Could you check a few things on this drawing? It's one solid part, dimensions in mm from its lowest x, y, z. A direction names the side the tool comes from. Coordinates: 2 decimals unless noted, no trailing zeros. Write each loop counter-clockwise with the first axis right and the second up, starting at its lowest first coordinate (ties: lowest second). Pieces come first, ordered by that corner, then holes.
Item 1: For the marked faces 4, 5 and 6, which set-ups out of +Z, -Z, +X, -X, +Y, -Y let a thin tool reach every point of the face, with its end or its side?
Item 2: If we mould it in two halves opening along Z, with no side actions, what happens to the marked faces 1, 2 and 3? For each: pulls with the +Z half, pulls with the -Z half, needs draft (parallel to the pull), parting line crosses it, or undercut.
Item 3: I want a section at C-C (x = 30). Please give me the cut outline in (y, z).
Item 4: I want a section at B-B (z = 7). Please give me the cut outline in (x, y).
Item 5: I want a section at D-D (x = 53). Please give me the cut outline in (y, z).
Item 6: Please list where these lines run through material, in increasing order: line 1 (Z direction, x = 7, y = 4); line 2 (X direction, y = 10.75, z = 30); line 3 (X direction, y = 7.75, z = 9).
Item 7: I want a section at A-A (y = 10). Please give me the cut outline in (x, z), and give its area (3 significant figures).
Item 8: I'm going to push flat-ended pins straight in: P1, Ø2, axis at y = 3.5, z = 18, coming from the -X side; P2, Ø4, axis at y = 13, z = 35.5, coming from the -X side; P3, Ø8.5, axis at x = 7, y = 10, coming from the +Z side; P4, Ø5, axis at x = 53, z = 25, coming from the +Y side. Where does each tip first touch, or does it pass through?
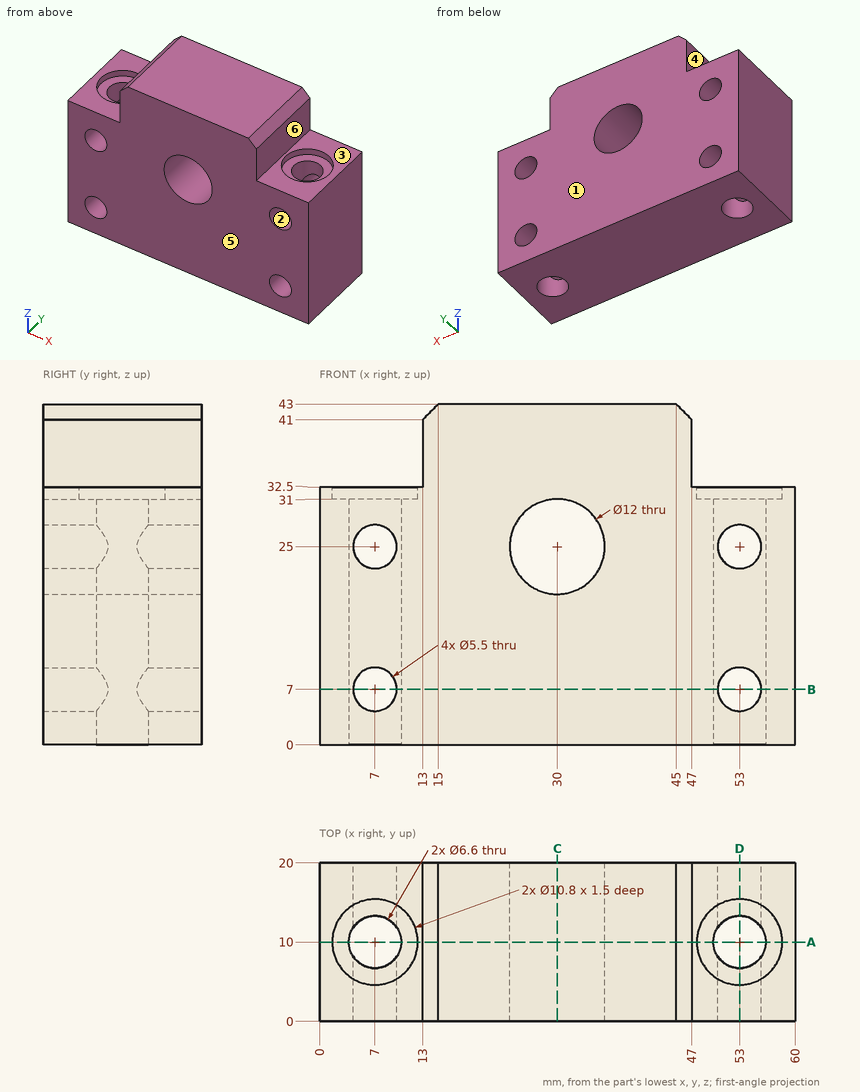
Answer:
1. face 4: +Z, -X, +Y, -Y
1. face 5: +Z, -Z, +X, -X, -Y
1. face 6: +Z, +X, +Y, -Y
2. face 1: needs draft
2. face 2: undercut
2. face 3: pulls with the +Z half
3. outline: (0, 0) - (20, 0) - (20, 19) - (0, 19) - close; (0, 31) - (20, 31) - (20, 43) - (0, 43) - close
4. outline: (0, 0) - (4.25, 0) - (4.25, 8.18) arc R3.3 cw to (4.25, 11.82) - (4.25, 20) - (0, 20) - close; (9.75, 0) - (50.25, 0) - (50.25, 8.18) arc R3.3 cw to (50.25, 11.82) - (50.25, 20) - (9.75, 20) - (9.75, 11.82) arc R3.3 cw to (9.75, 8.18) - close; (55.75, 0) - (60, 0) - (60, 20) - (55.75, 20) - (55.75, 11.82) arc R3.3 cw to (55.75, 8.18) - close
5. outline: (0, 0) - (6.7, 0) - (6.7, 4.25) - (0, 4.25) - close; (0, 9.75) - (6.7, 9.75) - (6.7, 22.25) - (0, 22.25) - close; (0, 27.75) - (6.7, 27.75) - (6.7, 31) - (4.6, 31) - (4.6, 32.5) - (0, 32.5) - close; (13.3, 0) - (20, 0) - (20, 4.25) - (13.3, 4.25) - close; (13.3, 9.75) - (20, 9.75) - (20, 22.25) - (13.3, 22.25) - close; (13.3, 27.75) - (20, 27.75) - (20, 32.5) - (15.4, 32.5) - (15.4, 31) - (13.3, 31) - close
6. line 1: z = 0 to 4.25, 9.75 to 22.25, 27.75 to 32.5
6. line 2: x = 0 to 3.79, 10.21 to 26.68, 33.32 to 49.79, 56.21 to 60
6. line 3: x = 0 to 4.59, 9.41 to 50.59, 55.41 to 60
7. outline: (0, 0) - (3.7, 0) - (3.7, 31) - (1.6, 31) - (1.6, 32.5) - (0, 32.5) - close; (10.3, 0) - (49.7, 0) - (49.7, 31) - (47.6, 31) - (47.6, 32.5) - (47, 32.5) - (47, 41) - (45, 43) - (15, 43) - (13, 41) - (13, 32.5) - (12.4, 32.5) - (12.4, 31) - (10.3, 31) - close; (56.3, 0) - (60, 0) - (60, 32.5) - (58.4, 32.5) - (58.4, 31) - (56.3, 31) - close; hole circle Ø12 at (30, 25)
7. area: 1,750 mm2
8. P1: stops at x = 0
8. P2: stops at x = 13
8. P3: stops at z = 31
8. P4: passes through
